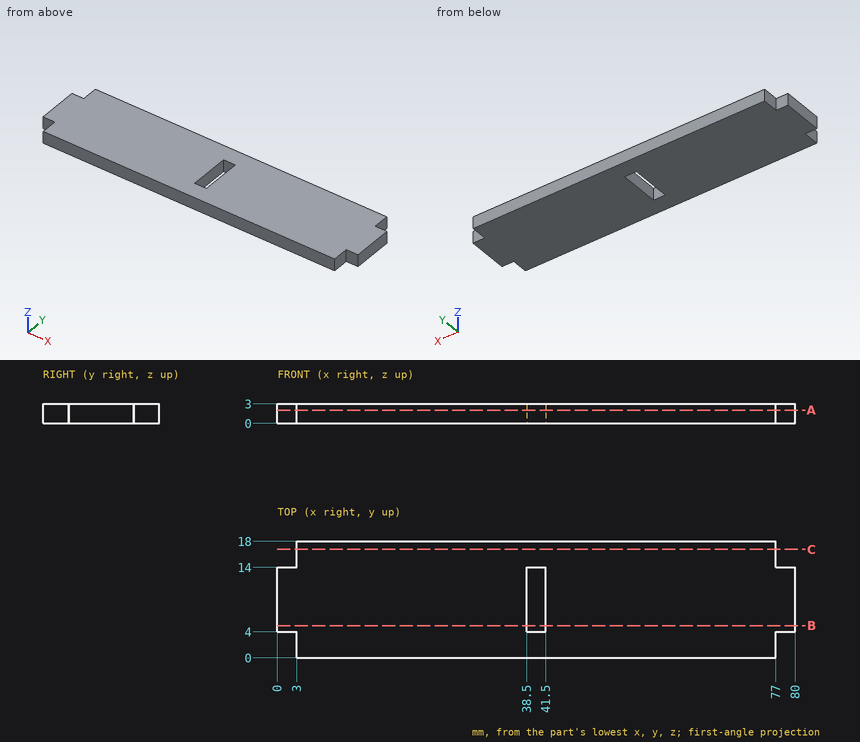
Source: three-view drawing plus pictorial views. Frame: mm from the lowest corner of the part. Give positions to 0.01 mm unless a question says otherwise; leave off trailing zeros. Loops run counter-clockwise (first coordinate to the right, second up) from the corner with the lowest first, then second, coordinate; pieces in that order, holes last. Notation, with made-up numbers: (51.25, 36) -> (72.25, 36) arc R15 cw to (72.25, 65) -> close; hole circle Ø5 at (70, 24.25). An arc over 180 degrees is marked (long way). Put each result on its own line as item: value. Start each with the question number.
1) Cut plane C-C (y = 16.75). Return loops of the section in (x, z).
2) Cut plane B-B (y = 5). Return loops of the section in (x, z), then the cut area to 3 significant figures.
3) Contact query for flat-ended pins moving along their axis: P1, Ø1.5, axis at y = 2, z = 2, coming from the -X side; P2, Ø1.5, axis at y = 1.5, z = 2, coming from the +X side; P3, Ø6, axis at x = 20, y = 3.5, coming from the -Z side; P4, Ø1.5, axis at x = 40.5, y = 6, coming from the -Z side. Output: stop coordinate, or through.
4) Cut plane A-A (z = 2.05). Return loops of the section in (x, y).
5) Material intervals for probe 1 along X at (y, z) = (11.5, 0.5); probe 2 along Y at (x, z) = (39, 2.5); probe 3 along X at (y, z) = (3.75, 0.85), sorted ascending.
Results are:
1. outline: (3, 0) -> (77, 0) -> (77, 3) -> (3, 3) -> close
2. outline: (0, 0) -> (38.5, 0) -> (38.5, 3) -> (0, 3) -> close; (41.5, 0) -> (80, 0) -> (80, 3) -> (41.5, 3) -> close
2. area: 231 mm2
3. P1: stops at x = 3
3. P2: stops at x = 77
3. P3: stops at z = 0
3. P4: passes through
4. outline: (0, 4) -> (3, 4) -> (3, 0) -> (77, 0) -> (77, 4) -> (80, 4) -> (80, 14) -> (77, 14) -> (77, 18) -> (3, 18) -> (3, 14) -> (0, 14) -> close; hole (38.5, 4) -> (41.5, 4) -> (41.5, 14) -> (38.5, 14) -> close
5. probe 1: x = 0 to 38.5, 41.5 to 80
5. probe 2: y = 0 to 4, 14 to 18
5. probe 3: x = 3 to 77
